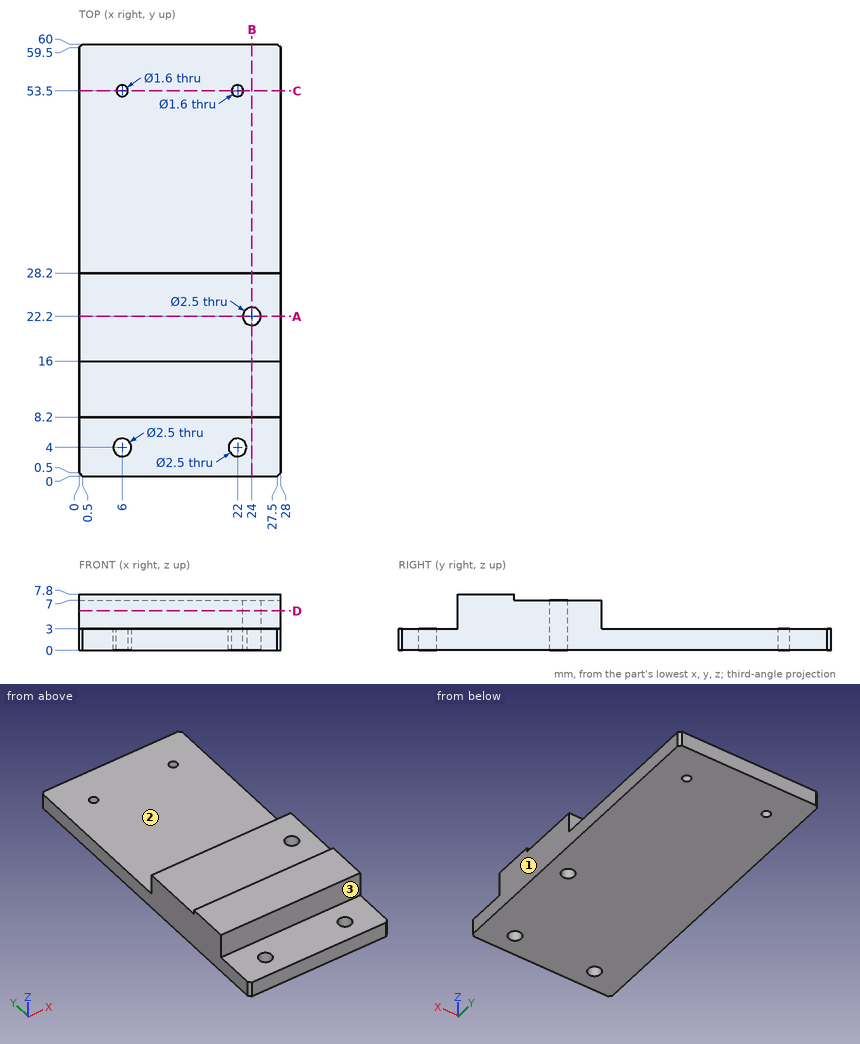
For this review, use the dimensioned drawing (mm, ordinates from the lowest corner) and the shaded views. A direction names the side the tool comes from. Round coordinates to 2 decimals unless told otherwise and drop trailing zeros. Order: outer loops, then holes, each group sorted by start corner. A loop starts at its lowest first (then second) coordinate and runs counter-clockwise, first axis right, second up. Notation, with made-up numbers: (60, 62) - (70, 62) arc R17 ccw to (70, 95) - close; hole circle Ø8 at (85.5, -26). An arc over 180 degrees is marked (long way). Use one line per item in the form item = value.
Q1. Clearance check with flat-ended pins moving along their axes: P1, Ø1, axis at x = 10, y = 7.5, coming from the -Z side; P2, Ø4, axis at x = 5.5, z = 7, coming from the -Y side; P3, Ø12, axis at x = 22, y = 23, coming from the +Z side; P4, Ø10, axis at x = 17, y = 37, coming from the +Z side. State where each tip first meets the part, or that it passes through.
Response values:
P1 = 0
P2 = 8.2
P3 = 7
P4 = 3
Q2. To check wall thickness, follow line 1 (X direction, y = 53.5, z = 1.25); line 2 (Y direction, x = 6, z = 0.75); line 3 (Y direction, x = 24, z = 2). State the ranges of each line that lie inside material, in increasing order.
Response values:
line_1 = 0 to 5.2, 6.8 to 21.2, 22.8 to 28
line_2 = 0 to 2.75, 5.25 to 52.7, 54.3 to 60
line_3 = 0 to 20.95, 23.45 to 60
Q3. Add section D-D on z = 5.5. Give the boundary of the cut face in (x, y).
Response values:
outline = (0, 8.2) - (28, 8.2) - (28, 28.2) - (0, 28.2) - close; hole circle Ø2.5 at (24, 22.2)
Q4. Add section A-A on y = 22.2. Give the boundary of the cut face in (x, z).
Response values:
outline = (0, 0) - (22.75, 0) - (22.75, 7) - (0, 7) - close; (25.25, 0) - (28, 0) - (28, 7) - (25.25, 7) - close
Q5. Add section B-B on x = 24. Give the boundary of the cut face in (y, z).
Response values:
outline = (0, 0) - (20.95, 0) - (20.95, 7) - (16, 7) - (16, 7.8) - (8.2, 7.8) - (8.2, 3) - (0, 3) - close; (23.45, 0) - (60, 0) - (60, 3) - (28.2, 3) - (28.2, 7) - (23.45, 7) - close
Q6. Add section C-C on y = 53.5. Give the boundary of the cut face in (x, z).
Response values:
outline = (0, 0) - (5.2, 0) - (5.2, 3) - (0, 3) - close; (6.8, 0) - (21.2, 0) - (21.2, 3) - (6.8, 3) - close; (22.8, 0) - (28, 0) - (28, 3) - (22.8, 3) - close
Q7. Tool access review of the marked faces 1, 2 and 3: name each direction out of +Z, -Z, +X, -X, +Y, -Y from which nothing blocks a thin tool from reaching the whole face with its end or side.
Response values:
face_1 = +Z, -Z, +X, +Y, -Y
face_2 = +Z, +X, -X, +Y
face_3 = +Z, +X, -X, -Y
